```python
from build123d import *

# Parameters (mm, degrees)
SKETCH1_R           = 7.15
SKETCH1_R_2         = 11
SKETCH1_W           = 50.4
SKETCH1_H           = 9.9
BOSS_EXTRUDE1_DEPTH = 9.5
M4_TAPPED_HOLE1_D   = 3.3


with BuildPart() as part:
    # Sketch1 → Boss-Extrude1 (new body)
    with BuildSketch(Plane(origin=(0, 0, 0), x_dir=(0, 0, -1), z_dir=(1, 0, 0))):
        Polygon((0, 0), (70, 0), (70, 135.667122158), (-64.5, 233.385504136), (-64.5, 368), (-134.5, 368), (-134.5, 208), align=None)
        with Locations((-99.5, 338)):
            Circle(SKETCH1_R, mode=Mode.SUBTRACT)
        with Locations((-99.5, 226)):
            Circle(SKETCH1_R, mode=Mode.SUBTRACT)
        with Locations((-103.5, 282)):
            Circle(SKETCH1_R_2, mode=Mode.SUBTRACT)
        Polygon((0, 18.416200794), (0, 100), (-99.5, 172.289806742), align=None, mode=Mode.SUBTRACT)
        with Locations((35, 15.05)):
            Rectangle(SKETCH1_W, SKETCH1_H, mode=Mode.SUBTRACT)
    extrude(amount=BOSS_EXTRUDE1_DEPTH)

    # M4 Tapped Hole1 (through all)
    with Locations(Plane(origin=(9.5, 0, 0), x_dir=(0, 0, -1), z_dir=(1, 0, 0))):
        with Locations((10, 34.7), (10, 52), (60, 34.7), (60, 52)):
            Hole(M4_TAPPED_HOLE1_D / 2)


solid = part.part
```
CAD build for the part. Positions are in the model's coordinates, mm. A direction names the side the tool comes from. Round coordinates to 2 decimals unless told otherwise and drop trailing zeros. Loops run counter-clockwise (first coordinate to the right, second up) from the corner with the lowest first, then second, coordinate; pieces in that order, holes last. Notation, with made-up numbers: M -36.75,60.25 L -22.75,60.25 A21 ccw -22.75,79.25 Z; hole C 8.5,-6 d7. An arc over 180 degrees is marked long. Return JSON: item names as keys, results as strings. Group by question number.
(1) Drop flat-ended pins along their axis: P1, Ø23, axis at y = 226, z = 99.5, coming from the +X side; P2, Ø5, axis at x = 6.5, z = -47.5, coming from the +Y side; P3, Ø3, axis at x = 7.5, z = -23, coming from the +Y side; P4, Ø13, axis at y = 338, z = 99.5, coming from the -X side. Give the stop position or say it passes through.
(2) Saw through at B-B, the plane x = 5. Give the number of separate pieces and of enclosed holes in the cut face, and give its area (3 significant figures).
(3) Mould opens along Z. For faces 1 (the flat face through (5, 67, -70)), 2 (the flat face through (5, 368, 99)), 3 (the cylindrical face through (4.68, 331.02, 101.05)) say: +Z half, -Z half, draft (parallel to the pull), parting line (faces both ways), or undercut.
(4) Tool access for faces 4 (the flat face through (5, 10.1, -35)), 5 (the flat face through (4.684, 105.456, 68.191)), 6 (the flat face through (5, 300, 64.5)): list every direction of +Z, -Z, +X, -X, +Y, -Y with a clear straight run to the whole face (end or side of a thin tool).
(5) Saw through at D-D, the plane y = 183. List the corners of the cut face in (x, z).
(6) Saw through at A-A, the plane y = 282. List the corners of the cut face in (x, z), and give its area (3 significant figures).
(7) Wall check: probe 1 along Z at (x, y) = (1.5, 51); probe 2 along Y at (x, z) = (4.5, -10); probe 3 along Z at (x, y) = (7, 347). Give the ranges that are in metal, low to high. Write a range as [from, to].
(8) Saw through at C-C, the plane z = 39.5. List the corners of the cut face in (x, y), and give its area (3 significant figures).
Answer list:
{
 "1": {"P1": "x = 9.5", "P2": "y = 153.83", "P3": "y = 170.9", "P4": "through"},
 "2": {"separate pieces": "1", "enclosed holes": "9", "area": "31,300 mm2"},
 "3": {"face 1": "-Z half", "face 2": "draft", "face 3": "undercut"},
 "4": {"face 4": "+X, -X", "face 5": "+Z, +X, -X, -Y", "face 6": "-Z, +X, -X, +Y"},
 "5": {"outline": "M 0,-4.85 L 9.5,-4.85 L 9.5,118.33 L 0,118.33 Z"},
 "6": {"outline": "M 0,64.5 L 9.5,64.5 L 9.5,92.5 L 0,92.5 Z; M 0,114.5 L 9.5,114.5 L 9.5,134.5 L 0,134.5 Z", "area": "456 mm2"},
 "7": {"probe 1": "[-70, -61.31], [-58.69, -11.31], [-8.69, 0], [21.07, 32.98]", "probe 2": "[0, 10.1], [20, 33.05], [36.35, 50.35], [53.65, 179.26]", "probe 3": "[64.5, 134.5]"},
 "8": {"outline": "M 0,61.09 L 9.5,61.09 L 9.5,79.5 L 0,79.5 Z; M 0,128.7 L 9.5,128.7 L 9.5,215.22 L 0,215.22 Z", "area": "997 mm2"}
}
